from build123d import *

# Parameters (mm, degrees)
SKETCH1_W           = 35.052
SKETCH1_H           = 35.052
SKETCH1_W_2         = 30.48
SKETCH1_H_2         = 30.48
BOSS_EXTRUDE1_DEPTH = 254
FILLET1_R           = 2
FILLET2_R           = 2
SKETCH2_R           = 12.7
CUT_EXTRUDE1_DEPTH  = 254
SKETCH3_R           = 3.81
CUT_EXTRUDE2_DEPTH  = 254
BOSS_EXTRUDE3_REACH = 37.052
SKETCH4_W           = 31.052
SKETCH4_H           = 5.462350323
SKETCH6_W           = 30.48
SKETCH6_H           = 30.48
SKETCH6_R           = 13
BOSS_EXTRUDE4_DEPTH = 217.402
SKETCH7_R           = 3.81
CUT_EXTRUDE3_DEPTH  = 217.402


with BuildPart() as part:
    # Sketch1 → Boss-Extrude1 (new body)
    with BuildSketch(Plane.XY):
        Rectangle(SKETCH1_W, SKETCH1_H)
        Rectangle(SKETCH1_W_2, SKETCH1_H_2, mode=Mode.SUBTRACT)
    extrude(amount=BOSS_EXTRUDE1_DEPTH)

    # Fillet1
    fillet1_edges = [part.edges().sort_by_distance(p)[0] for p in [
        (17.526, -17.526, 127),
        (-17.526, -17.526, 127),
        (-17.526, 17.526, 127),
        (17.526, 17.526, 127),
    ]]
    fillet(fillet1_edges, radius=FILLET1_R)

    # Fillet2
    fillet2_edges = [part.edges().sort_by_distance(p)[0] for p in [
        (15.24, -15.24, 127),
        (15.24, 15.24, 127),
        (-15.24, 15.24, 127),
        (-15.24, -15.24, 127),
    ]]
    fillet(fillet2_edges, radius=FILLET2_R)

    # Sketch2 → Cut-Extrude1 (cut)
    with BuildSketch(Plane.ZY.offset(17.526)):
        with Locations((20.234414068, 0)):
            Circle(SKETCH2_R)
    extrude(amount=-CUT_EXTRUDE1_DEPTH, mode=Mode.SUBTRACT)

    # Sketch3 → Cut-Extrude2 (cut)
    with BuildSketch(Plane(origin=(0, 17.526, 0), x_dir=(1, 0, 0), z_dir=(0, 1, 0))):
        with Locations((0, -135.527156181)):
            Circle(SKETCH3_R)
        with Locations((0, -216.910746369)):
            Circle(SKETCH3_R)
        with Locations((0, -71.490837775)):
            Circle(SKETCH3_R)
    extrude(amount=-CUT_EXTRUDE2_DEPTH, mode=Mode.SUBTRACT)

    # Sketch4 → Boss-Extrude3 (add, up to next)
    with BuildSketch(Plane(origin=(0, 17.526, 0), x_dir=(1, 0, 0), z_dir=(0, 1, 0)), mode=Mode.PRIVATE) as boss_extrude3_sk1:
        with Locations((0, -42.400785955)):
            Rectangle(SKETCH4_W, SKETCH4_H)
    boss_extrude3_tool1 = extrude(boss_extrude3_sk1.sketch, amount=-BOSS_EXTRUDE3_REACH, mode=Mode.PRIVATE) - part.part
    add(boss_extrude3_tool1.solids().sort_by_distance((0, 17.526, 42.400786))[0])

    # Sketch6 → Boss-Extrude4 (add)
    with BuildSketch(Plane.XY.offset(254)):
        Rectangle(SKETCH6_W, SKETCH6_H)
        Circle(SKETCH6_R, mode=Mode.SUBTRACT)
    extrude(amount=-BOSS_EXTRUDE4_DEPTH)

    # Sketch7 → Cut-Extrude3 (cut)
    with BuildSketch(Plane(origin=(0, 17.526, 0), x_dir=(1, 0, 0), z_dir=(0, 1, 0))):
        with Locations((0, -71.490837775)):
            Circle(SKETCH7_R)
        with Locations((0, -135.527156181)):
            Circle(SKETCH7_R)
        with Locations((0, -216.910746369)):
            Circle(SKETCH7_R)
    extrude(amount=-CUT_EXTRUDE3_DEPTH, mode=Mode.SUBTRACT)


solid = part.part
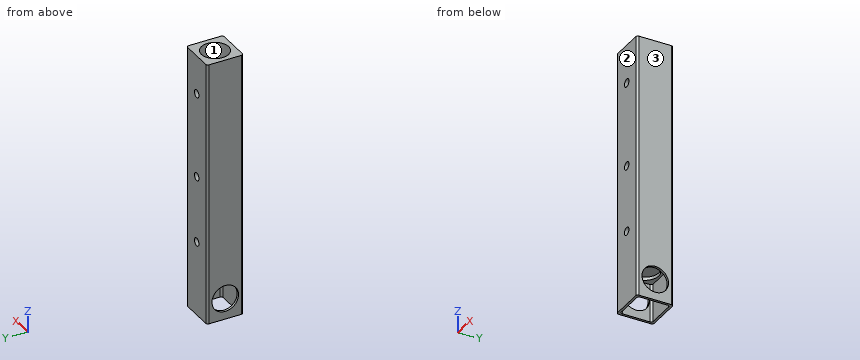
Work out the finished part from the listing and answer in its coordinate system (mm). Face numbers are marked on the shaded views. Round coordinates to 2 decimals unless told otherwise and drop trailing zeros. Write each loop counter-clockwise with the first axis right and the second up, starting at its lowest first coordinate (ties: lowest second). Pieces come first, ordered by that corner, then holes.
1) A cutting plane is placed at C-C (x = 0). Give the number of separate pieces and of enclosed holes in the cut face, plus the area to 3 significant figures.
2) A cutting plane is placed at B-B (z = 207). Give the vertices of the cut face in (x, y), plus the area to 3 significant figures.
3) Straight lines are drawn through the part: line 1 (Y direction, x = 0.5, z = 191); line 2 (Z direction, x = 0, y = -13.7); line 3 (Y direction, x = -3, z = 30.5). For each, find the intervals that lie inside material, in ascending order.
4) A cutting plane is placed at A-A (y = 0). Give the vertices of the cut face in (x, z), plus the area to 3 significant figures.
5) Given pin 1 Ø7 at (x, z) = (0, 135.53) entering from +Y; pin 2 Ø21 at (x, y) = (0, 0) entering from +Z; pin 3 Ø13 at (x, y) = (-2.5, -3) entering from -Z, each flat-ended and moving along its own axis, determine where each tip first touches the part or whether it passes through.
6) The mould has two halves that part along Y. Classify the marked faces 1, 2 and 3: pulls with the +Y half, pulls with the -Y half, needs draft (parallel to the pull), parting line crosses it, or undercut.
Completed:
1. separate pieces: 7
1. enclosed holes: 0
1. area: 2,070 mm2
2. outline: (-17.53, -15.53) arc R2 ccw to (-15.53, -17.53) - (15.53, -17.53) arc R2 ccw to (17.53, -15.53) - (17.53, 15.53) arc R2 ccw to (15.53, 17.53) - (-15.53, 17.53) arc R2 ccw to (-17.53, 15.53) - close; hole circle Ø26 at (0, 0)
2. area: 694 mm2
3. line 1: y = -17.53 to -12.99, 12.99 to 17.53
3. line 2: z = 36.6 to 67.68, 75.3 to 131.72, 139.34 to 213.1, 220.72 to 254
3. line 3: y = -17.53 to -15.24, 15.24 to 17.53
4. outline: (-17.53, 0) - (-15.24, 0) - (-15.24, 7.53) - (-17.53, 7.53) - close; (-17.53, 32.93) - (-15.24, 32.93) - (-15.24, 36.6) - (-13, 36.6) - (-13, 39.67) - (13, 39.67) - (13, 36.6) - (15.24, 36.6) - (15.24, 32.93) - (17.53, 32.93) - (17.53, 254) - (13, 254) - (13, 45.13) - (-13, 45.13) - (-13, 254) - (-17.53, 254) - close; (15.24, 0) - (17.53, 0) - (17.53, 7.53) - (15.24, 7.53) - close
4. area: 2,160 mm2
5. pin 1: passes through
5. pin 2: stops at z = 45.13
5. pin 3: stops at z = 39.67
6. face 1: undercut
6. face 2: pulls with the -Y half
6. face 3: needs draft
